Can you work these out from the model? Positions are in its coordinate system, mm. A direction names the side the tool comes from. Coordinates: 2 decimals unless noted, no trailing zeros. Loops run counter-clockwise (first coordinate to the right, second up) from the corner with the lowest first, then second, coordinate; pieces in that order, holes last. Notation, with made-up numbers: (74.25, 83) -> (102.25, 83) arc R28 cw to (102.25, 114) -> close; hole circle Ø7 at (-24.75, 4.5). An arc over 180 degrees is marked (long way). Put each result on its own line as item: value. Start each with the question number.
Item 1: If we section it at B-B on z = -2: Please give me the cut outline in (x, y), plus the area to 3 significant figures.
Item 2: If we section it at A-A on x = -30.5: Please give me the cut outline in (y, z), plus the area to 3 significant figures.
Item 3: If we section it at C-C on z = 33.5: Please give me the cut outline in (x, y).
Item 4: We'd pull the mould along X, two halves only. Please class faces 3 (the cylindrical face through (-30.235, -0.783, -23.183)), 4 (the cylindrical face through (-3.83, -19.566, -2.937)), 5 (the flat face through (-5, -39.688, -2)): pulls with the +X half, pulls with the -X half, needs draft (parallel to the pull), parting line crosses it, or undercut.
Item 5: If we section it at D-D on y = -14: Please give me the cut outline in (x, z), plus the area to 3 significant figures.
Item 6: For faces 1 (the cylindrical face through (12.35, -0.78, 10.08)), 2 (the cylindrical face through (-0.794, -20.371, 6.044)), which set-ups out of +Z, -Z, +X, -X, +Y, -Y let a thin tool reach every point of the face, with its end or its side?
Item 7: Will these pins go through, and if not, where does the flat tip stop? P1, Ø1.8, axis at x = 0.09, z = -34.65, coming from the -Y side; P2, Ø15, axis at x = 11.02, z = -22.88, coming from the -Y side.
Item 8: Please list where these lines run through material, in increasing order: L1, parallel to Z at x = 0, y = -26; L2, parallel to Y at x = 20, z = -18; L3, parallel to X at y = -29.5, z = -1. Write a range as from..to.
```python
from build123d import *

# Parameters (mm, degrees)
F0_R     = 38.1
F0_R_2   = 9.4615
F0_R_3   = 4.826
F1_DEPTH = 1.5875
F2_R     = 6.096
F2_R_2   = 4.826
F3_DEPTH = 38.1
F4_R     = 0.79375
F5_DEPTH = 282.448


with BuildPart() as f1:
    # F0 (on Front) → F1 (new body)
    with BuildSketch(Plane.XZ):
        Circle(F0_R)
        with Locations((-11.020647, -22.884609)):
            Circle(F0_R_2, mode=Mode.SUBTRACT)
        with Locations((-24.763169, -5.652032)):
            Circle(F0_R_2, mode=Mode.SUBTRACT)
        with Locations((11.020647, -22.884609)):
            Circle(F0_R_2, mode=Mode.SUBTRACT)
        with Locations((24.763169, -5.652032)):
            Circle(F0_R_2, mode=Mode.SUBTRACT)
        with Locations((-19.85852, 15.836641)):
            Circle(F0_R_2, mode=Mode.SUBTRACT)
        Circle(F0_R_3, mode=Mode.SUBTRACT)
        with Locations((19.85852, 15.836641)):
            Circle(F0_R_2, mode=Mode.SUBTRACT)
        with Locations((0, 25.4)):
            Circle(F0_R_2, mode=Mode.SUBTRACT)
    extrude(amount=F1_DEPTH)

    # F2 (on face) → F3 (join)
    with BuildSketch(Plane.XZ.offset(1.5875)):
        Circle(F2_R)
        Circle(F2_R_2, mode=Mode.SUBTRACT)
    extrude(amount=F3_DEPTH)

    # F4 (on face) → F5 (cut)
    with BuildSketch(Plane.XZ.offset(1.5875)):
        with BuildLine():
            ThreePointArc((0.79375, -6.88975), (0.561266, -6.328484), (0, -6.096))
            ThreePointArc((0, -6.096), (-0.561266, -7.451016), (0.79375, -6.88975))
        make_face()
        with BuildLine():
            ThreePointArc((6.096, 0), (6.88975, -0.79375), (7.6835, 0))
            ThreePointArc((7.6835, 0), (6.88975, 0.79375), (6.096, 0))
        make_face()
        with Locations((27.146798, -21.533931)):
            Circle(F4_R)
        with Locations((33.761657, 7.798035)):
            Circle(F4_R)
        with Locations((0.089846, -34.650408)):
            Circle(F4_R)
        with Locations((-27.034762, -21.674421)):
            Circle(F4_R)
        with Locations((-33.801643, 7.622847)):
            Circle(F4_R)
        with Locations((-15.115198, 31.179956)):
            Circle(F4_R)
        with Locations((14.9533, 31.257922)):
            Circle(F4_R)
        with BuildLine():
            ThreePointArc((0.79375, 6.88975), (-0.561266, 7.451016), (0, 6.096))
            ThreePointArc((0, 6.096), (0.561266, 6.328484), (0.79375, 6.88975))
        make_face()
        with Locations((-6.88975, 0)):
            Circle(F4_R)
    extrude(amount=-F5_DEPTH, mode=Mode.SUBTRACT)


solid = f1.part
```
Solutions:
1. outline: (-38.05, -1.59) -> (-33.49, -1.59) -> (-33.49, 0) -> (-38.05, 0) -> close; (-16.03, -1.59) -> (-5.76, -1.59) -> (-5.76, -39.69) -> (-4.39, -39.69) -> (-4.39, 0) -> (-16.03, 0) -> close; (4.39, -39.69) -> (5.76, -39.69) -> (5.76, -1.59) -> (16.03, -1.59) -> (16.03, 0) -> (4.39, 0) -> close; (33.49, -1.59) -> (38.05, -1.59) -> (38.05, 0) -> (33.49, 0) -> close
1. area: 156 mm^2
2. outline: (-1.59, -22.83) -> (0, -22.83) -> (0, -13.18) -> (-1.59, -13.18) -> close; (-1.59, 1.87) -> (0, 1.87) -> (0, 22.83) -> (-1.59, 22.83) -> close
2. area: 48.6 mm^2
3. outline: (-18.15, -1.59) -> (-4.89, -1.59) -> (-4.89, 0) -> (-18.15, 0) -> close; (4.89, -1.59) -> (18.15, -1.59) -> (18.15, 0) -> (4.89, 0) -> close
4. face 3: parting line crosses it
4. face 4: undercut
4. face 5: needs draft
5. outline: circle Ø12.19 at (0, 0); hole circle Ø9.65 at (0, 0)
5. area: 43.6 mm^2
6. face 1: +Y, -Y
6. face 2: -Y
7. P1: y = -1.59
7. P2: through
8. L1: -6.1..-4.83, 4.83..6.1
8. L2: -1.59..0
8. L3: -6.01..-4.72, 4.72..6.01
